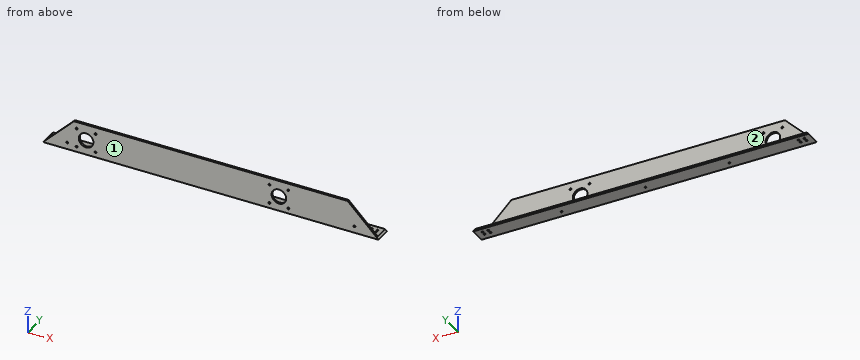
from build123d import *

# Parameters (mm, degrees)
BOSS_EXTRUDE1_DEPTH              = 550
CHAMFER7_SIZE                    = 50.8
CHAMFER8_SIZE                    = 50.8
BOTTHOMHOLES_SKETCH2_R           = 12
BOTTHOMHOLES_SKETCH2_R_2         = 1.5875
BOTTOMHOLES_CUT_EXTRUDE1_DEPTH   = 553.788015993
LEFTSIDEHOLES_SKETCH3_R          = 1.5875
LEFTSIDEHOLES_CUT_EXTRUDE2_DEPTH = 553.924768843


with BuildPart() as part:
    # Sketch1 → Boss-Extrude1 (new body)
    with BuildSketch(Plane(origin=(0, 0, 0), x_dir=(0, 0, -1), z_dir=(1, 0, 0))):
        Polygon((0, 0), (-50.8, 0), (-50.8, 3.175), (-3.175, 3.175), (-3.175, 25.4), (0, 25.4), align=None)
    extrude(amount=BOSS_EXTRUDE1_DEPTH)

    # Chamfer7
    chamfer7_edges = [part.edges().sort_by_distance(p)[0] for p in [
        (0, 1.5875, 50.8),
    ]]
    chamfer(chamfer7_edges, length=CHAMFER7_SIZE - 0.0001)  # a hair under: the kernel refuses the full size

    # Chamfer8
    chamfer8_edges = [part.edges().sort_by_distance(p)[0] for p in [
        (550, 1.5875, 50.8),
    ]]
    chamfer(chamfer8_edges, length=CHAMFER8_SIZE - 0.0001)  # a hair under: the kernel refuses the full size

    # BotthomHoles-Sketch2 → BottomHoles-Cut-Extrude1 (cut, through all)
    with BuildSketch(Plane(origin=(0, 3.175, 0), x_dir=(1, 0, 0), z_dir=(0, 1, 0))):
        with Locations(Location((70.575, -24.175, 0), (0, 0, 270))):
            Circle(BOTTHOMHOLES_SKETCH2_R)
        with Locations(Location((386.575, -24.175, 0), (0, 0, 270))):
            Circle(BOTTHOMHOLES_SKETCH2_R)
        with Locations(Location((55.075, -8.675, 0), (0, 0, 270))):
            Circle(BOTTHOMHOLES_SKETCH2_R_2)
        with Locations(Location((86.075, -8.675, 0), (0, 0, 270))):
            Circle(BOTTHOMHOLES_SKETCH2_R_2)
        with Locations(Location((371.075, -8.675, 0), (0, 0, 270))):
            Circle(BOTTHOMHOLES_SKETCH2_R_2)
        with Locations(Location((402.075, -8.675, 0), (0, 0, 270))):
            Circle(BOTTHOMHOLES_SKETCH2_R_2)
        with Locations(Location((55.075, -39.675, 0), (0, 0, 270))):
            Circle(BOTTHOMHOLES_SKETCH2_R_2)
        with Locations(Location((86.075, -39.675, 0), (0, 0, 270))):
            Circle(BOTTHOMHOLES_SKETCH2_R_2)
        with Locations(Location((371.075, -39.675, 0), (0, 0, 270))):
            Circle(BOTTHOMHOLES_SKETCH2_R_2)
        with Locations(Location((402.075, -39.675, 0), (0, 0, 270))):
            Circle(BOTTHOMHOLES_SKETCH2_R_2)
        with Locations(Location((39.6875, -11.1125, 0), (0, 0, 270))):
            Circle(BOTTHOMHOLES_SKETCH2_R_2)
        with Locations(Location((510.3125, -11.1125, 0), (0, 0, 270))):
            Circle(BOTTHOMHOLES_SKETCH2_R_2)
    extrude(amount=-BOTTOMHOLES_CUT_EXTRUDE1_DEPTH, mode=Mode.SUBTRACT)

    # LeftSideHoles-Sketch3 → LeftSideHoles-Cut-Extrude2 (cut, through all)
    with BuildSketch(Plane(origin=(0, 0, 0), x_dir=(-1, 0, 0), z_dir=(0, 0, -1))):
        with Locations(Location((-538.8875, 17.4625, 0), (0, 0, 90))):
            Circle(LEFTSIDEHOLES_SKETCH3_R)
        with Locations(Location((-529.3625, 17.4625, 0), (0, 0, 90))):
            Circle(LEFTSIDEHOLES_SKETCH3_R)
        with Locations(Location((-538.8875, 11.1125, 0), (0, 0, 90))):
            Circle(LEFTSIDEHOLES_SKETCH3_R)
        with Locations(Location((-529.3625, 11.1125, 0), (0, 0, 90))):
            Circle(LEFTSIDEHOLES_SKETCH3_R)
        with Locations(Location((-11.1125, 11.1125, 0), (0, 0, 90))):
            Circle(LEFTSIDEHOLES_SKETCH3_R)
        with Locations(Location((-20.6375, 11.1125, 0), (0, 0, 90))):
            Circle(LEFTSIDEHOLES_SKETCH3_R)
        with Locations(Location((-20.6375, 17.4625, 0), (0, 0, 90))):
            Circle(LEFTSIDEHOLES_SKETCH3_R)
        with Locations(Location((-11.1125, 17.4625, 0), (0, 0, 90))):
            Circle(LEFTSIDEHOLES_SKETCH3_R)
        with Locations(Location((-412.5, 11.1125, 0), (0, 0, 90))):
            Circle(LEFTSIDEHOLES_SKETCH3_R)
        with Locations(Location((-275, 11.1125, 0), (0, 0, 90))):
            Circle(LEFTSIDEHOLES_SKETCH3_R)
        with Locations(Location((-137.5, 11.1125, 0), (0, 0, 90))):
            Circle(LEFTSIDEHOLES_SKETCH3_R)
    extrude(amount=-LEFTSIDEHOLES_CUT_EXTRUDE2_DEPTH, mode=Mode.SUBTRACT)


solid = part.part
The model under review builds one solid part; all positions refer to its coordinate system, in mm. Face numbers are marked on the shaded views. A direction names the side the tool comes from. Round coordinates to 2 decimals unless told otherwise and drop trailing zeros. Order: outer loops, then holes, each group sorted by start corner. A loop starts at its lowest first (then second) coordinate and runs counter-clockwise, first axis right, second up. Notation, with made-up numbers: (84.25, 64.5) -> (106.25, 64.5) arc R16 cw to (106.25, 78.5) -> close; hole circle Ø6 at (23, 22). An arc over 180 degrees is marked (long way). Return JSON: item names as keys, results as strings.
1. Take a section at A-A (z = 27.5). Write out the cut boundary in (x, y) (3 decimals), then the cut area to 3 significant figures.
Answer block:
{"outline": "(27.5, 0) -> (59.045, 0) -> (59.045, 3.175) -> (27.5, 3.175) -> close; (82.105, 0) -> (375.045, 0) -> (375.045, 3.175) -> (82.105, 3.175) -> close; (398.105, 0) -> (522.5, 0) -> (522.5, 3.175) -> (398.105, 3.175) -> close", "area": "1,430 mm²"}
2. Insertion check: P1, Ø4, axis at x = 11.11, y = 11.11, coming from the +Z side (3 decimals); P2, Ø3, axis at x = 129.5, z = 19, coming from the +Y side (3 decimals); P3, Ø5, axis at y = 5, z = 7.5, coming from the -X side. Each pin has a flat end and moves straight along its axis. Give the tip position at first contact, or say it passes through.
Answer block:
{"P1": "stops at z = 3.175", "P2": "stops at y = 3.175", "P3": "stops at x = 5.79"}
3. Take a section at B-B (x = 421). Write out the cut boundary in (y, z) (3 decimals), then the cut area to 3 significant figures.
Answer block:
{"outline": "(0, 0) -> (25.4, 0) -> (25.4, 3.175) -> (3.175, 3.175) -> (3.175, 50.8) -> (0, 50.8) -> close", "area": "232 mm²"}
4. For the marked faces 1 and 2, list the 3-axis set-ups (+Z, -Z, +X, -X, +Y, -Y) from which the entire face can be reached by the end or side of a thin tool; tool diameter is ignored.
Answer block:
{"face 1": "+Z, -Z, +X, -X, -Y", "face 2": "+Z, +X, -X, +Y"}
5. For L1, parallel to Y at x = 379, z = 42 (3 decimals), list the stretches that pass through material, from the lowest coordinate up. Write a range as [from, to].
Answer block:
{"L1": "y = [0, 3.175]"}
